Input: part model. Units: mm. Frame: model coordinates. Face numbers are marked on the shaded views. Coordinates: 2 decimals unless noted, no trailing zeros. Loops run counter-clockwise (first coordinate to the right, second up) from the corner with the lowest first, then second, coordinate; pieces in that order, holes last.
Item 1: Contact query for a flat-ended pin moving along its axis: P1, Ø1, axis at x = -1, z = -13.5, coming from the +Y side. Output: stop coordinate, or through.
Item 2: Section C-C on z = -16.25. Return loops of the section in (x, y) (3 decimals), and give its area (3 significant figures).
Item 3: Section A-A on z = -3.5. Return loops of the section in (x, y), and give its area (3 significant figures).
Item 4: Section B-B on y = 0.1. Return loops of the section in (x, z).
Item 5: Pull-direction query (X, two-part tool) for the marked faces 1 and 2; classes: released by +X, released by -X, zero draft, split by the parting line, or undercut.
Item 6: Ray query, line 1 along X through (y, z) = (0.1, 0); line 2 along Z through (x, y) = (-0.3, 0.1); line 3 along Z through (x, y) = (-0.05, 0.1). Return the intervals inside material, ascending.
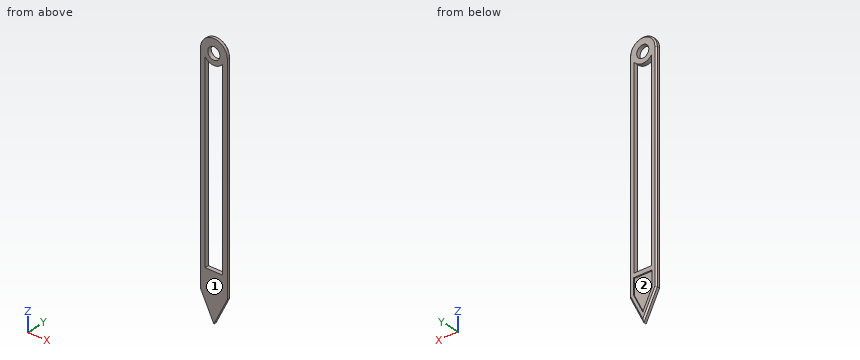
```python
from build123d import *

# Parameters (mm, degrees)
SKETCH1_R           = 0.45
BOSS_EXTRUDE1_DEPTH = 0.3
CUT_EXTRUDE1_DEPTH  = 0.1
CHAMFER1_SIZE       = 0.1


with BuildPart() as part:
    # Sketch1 → Boss-Extrude1 (new body)
    with BuildSketch(Plane(origin=(0, 0, 0), x_dir=(1, 0, 0), z_dir=(0, 1, 0))):
        with BuildLine():
            Line((-1, 0), (-1, 16))
            Line((-1, 16), (0, 18))
            Line((0, 18), (1, 16))
            Line((1, 16), (1, 0))
            ThreePointArc((1, 0), (0, -1), (-1, 0))
        make_face()
        Circle(SKETCH1_R, mode=Mode.SUBTRACT)
        with BuildLine():
            Line((-0.65, 0.466368953), (-0.65, 14.5))
            Line((-0.65, 14.5), (0.65, 14.5))
            Line((0.65, 14.5), (0.65, 0.466368953))
            ThreePointArc((0.65, 0.466368953), (0, 0.8), (-0.65, 0.466368953))
        make_face(mode=Mode.SUBTRACT)
    extrude(amount=BOSS_EXTRUDE1_DEPTH)

    # Sketch2 → Cut-Extrude1 (cut)
    with BuildSketch(Plane(origin=(0, 0.3, 0), x_dir=(1, 0, 0), z_dir=(0, 1, 0))):
        Polygon((-0.7, 15.929179607), (-0.7, 14.8), (0.7, 14.8), (0.7, 15.929179607), (0, 17.329179607), align=None)
    extrude(amount=-CUT_EXTRUDE1_DEPTH, mode=Mode.SUBTRACT)

    # Chamfer1
    chamfer1_edges = [part.edges().sort_by_distance(p)[0] for p in [
        (0.5, 0.3, -17),
        (-0.5, 0.3, -17),
        (-1, 0.3, -8),
        (0, 0.3, 1),
        (1, 0.3, -8),
    ]]
    chamfer(chamfer1_edges, length=CHAMFER1_SIZE)


solid = part.part
```
Results found:
1. P1: stops at y = 0.3
2. outline: (-0.875, 0) - (0.875, 0) - (0.875, 0.2) - (0.763, 0.3) - (0.54, 0.3) - (0.54, 0.2) - (-0.54, 0.2) - (-0.54, 0.3) - (-0.763, 0.3) - (-0.875, 0.2) - close
2. area: 0.406 mm2
3. outline: (-1, 0) - (-0.65, 0) - (-0.65, 0.3) - (-0.9, 0.3) - (-1, 0.2) - close; (0.65, 0) - (1, 0) - (1, 0.2) - (0.9, 0.3) - (0.65, 0.3) - close
3. area: 0.200 mm2
4. outline: (-1, -16) - (0, -18) - (1, -16) - (1, 0) arc R1 ccw to (-1, 0) - close; hole (-0.65, -14.5) - (0.65, -14.5) - (0.65, -0.47) arc R0.8 cw to (-0.65, -0.47) - close; hole circle Ø0.9 at (0, 0)
5. face 1: zero draft
5. face 2: undercut
6. line 1: x = -1 to -0.45, 0.45 to 1
6. line 2: z = -17.4 to -14.5, -0.74 to -0.34, 0.34 to 0.95
6. line 3: z = -17.9 to -14.5, -0.8 to -0.45, 0.45 to 1
